from build123d import *

# Parameters (mm, degrees)
SKETCH1_R           = 0.635
BOSS_EXTRUDE1_DEPTH = 5.08
BOSS_EXTRUDE2_DEPTH = 1.27
BOSS_EXTRUDE3_DEPTH = 27.94
CHAMFER1_SIZE       = 1.016
BOSS_EXTRUDE4_DEPTH = 7.112
CUT_EXTRUDE1_REACH  = 95.615
FILLET1_R           = 11.43
FILLET2_R           = 0.508
BOSS_EXTRUDE5_DEPTH = 6.35
SKETCH10_W          = 38.1
SKETCH10_H          = 0.635
SKETCH10_H_2        = 1.27
CUT_EXTRUDE2_DEPTH  = 5.08


# Some blends are built 0.0001 mm under size
with BuildPart() as part:
    # Sketch1 → Boss-Extrude1 (new, symmetric)
    with BuildSketch(Plane(origin=(0, 0, 0), x_dir=(0, 0, -1), z_dir=(1, 0, 0))):
        Circle(SKETCH1_R)
    extrude(amount=BOSS_EXTRUDE1_DEPTH, both=True)

    # Sketch2 → Boss-Extrude2 (add)
    with BuildSketch(Plane(origin=(5.08, 0, 0), x_dir=(0, 0, -1), z_dir=(1, 0, 0))):
        with BuildLine():
            Line((0, 1.016), (6.35, 1.016))
            Line((6.35, 1.016), (6.35, -1.016))
            Line((6.35, -1.016), (0, -1.016))
            ThreePointArc((0, -1.016), (-1.016, 0), (0, 1.016))
        make_face()
    boss_extrude2 = extrude(amount=BOSS_EXTRUDE2_DEPTH)

    # Mirror1: Boss-Extrude2 across plane
    add(boss_extrude2.mirror(Plane(origin=(0, 0, 0), x_dir=(0, 0, 1), z_dir=(1, 0, 0))))

    # Sketch4 → Boss-Extrude3 (add, symmetric)
    with BuildSketch(Plane(origin=(0, 0, 0), x_dir=(0, 0, -1), z_dir=(1, 0, 0))):
        Polygon((2.032, 1.016), (2.032, 0), (89.3191, 0), (89.3191, 1.27), (2.413, 1.27), align=None)
    extrude(amount=BOSS_EXTRUDE3_DEPTH, both=True)

    # Chamfer1
    chamfer1_edges = [part.edges().sort_by_distance(p)[0] for p in [
        (-27.94, 1.27, -45.86605),
        (27.94, 1.27, -45.86605),
    ]]
    chamfer(chamfer1_edges, length=CHAMFER1_SIZE)

    # Sketch5 → Boss-Extrude4 (add)
    with BuildSketch(Plane.XY.offset(-2.032)):
        Polygon((6.35, 1.016), (27.178, 1.016), (27.94, 0.254), (27.94, 0), (27.178, 0), (6.35, 0), align=None)
        Polygon((-27.94, 0), (-27.178, 0), (-6.35, 0), (-6.35, 1.016), (-27.178, 1.016), (-27.94, 0.254), align=None)
    extrude(amount=BOSS_EXTRUDE4_DEPTH)

    # Sketch6 → Cut-Extrude1 (cut, up to next)
    with BuildSketch(Plane(origin=(0, 1.27, 0), x_dir=(1, 0, 0), z_dir=(0, 1, 0)), mode=Mode.PRIVATE) as cut_extrude1_sk1:
        with BuildLine():
            Line((24.13, -3.556), (6.35, -3.556))
            Line((6.35, -3.556), (6.35, -5.08))
            Line((6.35, -5.08), (27.94, -5.08))
            Line((27.94, -5.08), (27.94, 5.461))
            ThreePointArc((27.94, 5.461), (25.86406568, 1.919644773), (25.4, -2.159))
            ThreePointArc((25.4, -2.159), (25.073995365, -3.138404878), (24.13, -3.556))
        make_face()
    cut_extrude1_tool1 = extrude(cut_extrude1_sk1.sketch, amount=-CUT_EXTRUDE1_REACH, mode=Mode.PRIVATE) & part.part
    # Sketch6 → Cut-Extrude1 (cut, up to next)
    with BuildSketch(Plane(origin=(0, 1.27, 0), x_dir=(1, 0, 0), z_dir=(0, 1, 0)), mode=Mode.PRIVATE) as cut_extrude1_sk2:
        with BuildLine():
            Line((-27.94, -5.08), (-27.94, 5.461))
            ThreePointArc((-27.94, 5.461), (-25.86406568, 1.919644773), (-25.4, -2.159))
            ThreePointArc((-25.4, -2.159), (-25.073995365, -3.138404878), (-24.13, -3.556))
            Line((-24.13, -3.556), (-6.35, -3.556))
            Line((-6.35, -3.556), (-6.35, -5.08))
            Line((-6.35, -5.08), (-27.94, -5.08))
        make_face()
    cut_extrude1_tool2 = extrude(cut_extrude1_sk2.sketch, amount=-CUT_EXTRUDE1_REACH, mode=Mode.PRIVATE) & part.part
    add(cut_extrude1_tool1.solids().sort_by_distance((26.091995, 1.27, -1.843668))[0], mode=Mode.SUBTRACT)
    add(cut_extrude1_tool2.solids().sort_by_distance((-27.699742, 1.27, -0.1905))[0], mode=Mode.SUBTRACT)

    # Fillet1
    # the kernel refuses this fillet: 11.43 mm, written as the material it adds along each edge
    with BuildSketch(Plane(origin=(5.08, 1.016, -2.032), x_dir=(0, 0.5547001962252287, -0.832050294337844), z_dir=(1, 0, 0))) as fillet1_piece_1_section:
        with BuildLine():
            CenterArc((4.663449523, 10.628184011), FILLET1_R, 236.309932474, 12.101492032)
            Line((-1.676773719, 1.117849146), (0, 0))
            Line((0, 0), (0.457905012, 0))
        make_face()
    fillet1_piece_1 = extrude(amount=25.860343839, mode=Mode.PRIVATE)
    fillet1_piece_1 = fillet1_piece_1 - Plane(origin=(35.272791519, 1.208479731, 1.216597173), x_dir=(-0.7393665158371048, 0, -0.6733031674208139), z_dir=(0, 1, 0)) * Cylinder(9.917667845, 59, mode=Mode.PRIVATE)
    add(fillet1_piece_1)
    with BuildSketch(Plane(origin=(-30.940343839, 1.016, -2.032), x_dir=(0, 0.5547001962260483, -0.8320502943372975), z_dir=(1, 0, 0))) as fillet1_piece_2_section:
        with BuildLine():
            CenterArc((4.663449523, 10.628184011), FILLET1_R, 236.309932474, 12.101492032)
            Line((-1.676773719, 1.117849146), (0, 0))
            Line((0, 0), (0.457905012, 0))
        make_face()
    fillet1_piece_2 = extrude(amount=25.860343839, mode=Mode.PRIVATE)
    fillet1_piece_2 = fillet1_piece_2 - Plane(origin=(-35.272791519, 1.208479731, 1.216597173), x_dir=(0.7393665158371048, 0, -0.6733031674208138), z_dir=(0, 1, 0)) * Cylinder(9.917667845, 59, mode=Mode.PRIVATE)
    add(fillet1_piece_2)

    # Fillet2
    fillet2_edges = [part.edges().sort_by_distance(p)[0] for p in [
        (-25.86406568, 0, -1.919644773),
        (-15.24, 0, 3.556),
        (-25.669565682, 1.08391662, -1.260939708),
        (-25.356203761, 1.016, 1.070232197),
        (-15.24, 1.016, 3.556),
        (25.86406568, 0, -1.919644773),
        (25.073995365, 0, 3.138404878),
        (25.669564301, 1.083916034, -1.260934355),
        (25.356203761, 1.016, 1.070232197),
        (25.073995365, 1.016, 3.138404878),
        (-25.073995365, 0, 3.138404878),
        (-25.073995365, 1.016, 3.138404878),
        (15.24, 0, 3.556),
        (15.24, 1.016, 3.556),
    ]]
    fillet(fillet2_edges, radius=FILLET2_R - 0.0001)  # a hair under: the kernel refuses the full size

    # Sweep1: sweep along a path in Sketch8
    with BuildLine(Plane(origin=(0, 0, 0), x_dir=(0, 0, -1), z_dir=(1, 0, 0))) as sweep1_path:
        ThreePointArc((89.3191, 0), (107.756716577, -1.34549632), (125.80366, -5.35347567))
    # Sketch7 → Sweep1 (sweep)
    with BuildSketch(Plane(origin=(0, 0, -89.3191), x_dir=(-1, 0, 0), z_dir=(0, 0, -1))):
        Polygon((-27.94, 0), (-27.94, 0.254), (-26.924, 1.27), (26.924, 1.27), (27.94, 0.254), (27.94, 0), align=None)
    sweep(path=sweep1_path.line)

    # Sketch9 → Boss-Extrude5 (add)
    with BuildSketch(Plane(origin=(0, -35.059237678, -116.894226193), x_dir=(-1, 0, 0), z_dir=(0, -0.28728000000000004, -0.957846648268918))):
        Polygon((-27.94, 31.013066718), (-27.94, 31.267066718), (-26.924, 32.283066718), (26.924, 32.283066718), (27.94, 31.267066718), (27.94, 31.013066718), align=None)
    extrude(amount=BOSS_EXTRUDE5_DEPTH)

    # Sketch10 → Cut-Extrude2 (cut)
    with BuildSketch(Plane(origin=(0, -36.883465678, -122.97655241), x_dir=(-1, 0, 0), z_dir=(0, -0.28727999999993675, -0.9578466482689367))):
        with Locations((0, 31.719186718)):
            Rectangle(SKETCH10_W, SKETCH10_H)
        with Locations((0, 30.449186718)):
            Rectangle(SKETCH10_W, SKETCH10_H_2)
    extrude(amount=-CUT_EXTRUDE2_DEPTH, mode=Mode.SUBTRACT)


solid = part.part
For this review, take the finished solid that the model builds, in its own axes (mm). A direction names the side the tool comes from. Give positions to 0.01 mm unless a question says otherwise; leave off trailing zeros. Order: outer loops, then holes, each group sorted by start corner. A loop starts at its lowest first (then second) coordinate and runs counter-clockwise, first axis right, second up. Notation, with made-up numbers: (51.5, 67) -> (110.5, 67) arc R16 cw to (110.5, 73) -> close; hole circle Ø1 at (-16, -36.5). An arc over 180 degrees is marked (long way). Write item = value, one per line.
1) For faces 4 (the face through (0.267, -6.086, -129.599)), 5 (the face through (-27.65, -0.77, -107.58)), 6 (the face through (15, 1.016, 1)), list the 3-axis set-ups (+Z, -Z, +X, -X, +Y, -Y) from which the entire face can be reached by the end or side of a thin tool; tool diameter is ignored.
Findings:
face_4 = none
face_5 = -Z, -X, +Y
face_6 = +Z, +X, -X, +Y
2) Draft analysis for pull direction Z (two halves, no side actions). For faces 1 (the face through (-0.391, -5.645, -126.775)), 2 (the face through (5.08, -0.2, -2.4)), 3 (the face through (-15, 1.016, 2)), state which applies: pulls with the +Z half, pulls with the -Z half, needs draft (parallel to the pull), parting line crosses it, or undercut.
Findings:
face_1 = pulls with the +Z half
face_2 = undercut
face_3 = needs draft
3) We need section C-C, the plane z = -39.5. Give the boundary of the cut face in (x, y), and give its area (3 significant figures).
Findings:
outline = (-27.94, 0) -> (27.94, 0) -> (27.94, 0.25) -> (26.92, 1.27) -> (-26.92, 1.27) -> (-27.94, 0.25) -> close
area = 69.9 mm^2
4) Insertion check: pin 1 (2 mm diameter, centred on x = 8, z = -88.5, fed in from -Y); pin 2 (0.9 mm diameter, centred on x = 14.5, z = 1, fed in from +Y); pin 3 (10 mm diameter, centred on x = 7, z = -95, fed in from +Y). Each pin has a flat end and moves straight along its axis. Give the tip position at first contact, or say it passes through.
Findings:
pin_1 = 0
pin_2 = 1.02
pin_3 = 1.27
5) To check wall thickness, follow L1, parallel to X at y = 0.5, z = -30.5; L2, parallel to Y at x = -5.5, z = -16; L3, parallel to Y at x = -6, z = -98.5. State the ranges of each line that lie inside material, in increasing order. Write a range as from..to.
Findings:
L1 = -27.69..27.69
L2 = 0..1.27
L3 = -0.33..0.94
